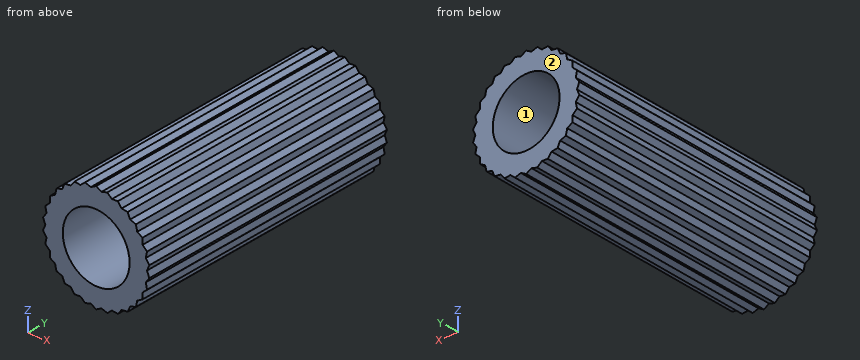
```python
from build123d import *

# Parameters (mm, degrees)
SKETCH_1_R      = 1
EXTRUDE_1_DEPTH = 8


with BuildPart() as part:
    # 草图1 → 凸台-拉伸1 (new body)
    with BuildSketch(Plane(origin=(0, 0, 0), x_dir=(1, 0, 0), z_dir=(0, 1, 0))):
        Polygon((0, 1.6), (-0.158843146, 1.511291584), (-0.332658705, 1.565036161), (-0.469587231, 1.44524089), (-0.650778629, 1.461672732), (-0.7598081, 1.316026234), (-0.940456404, 1.294427191), (-1.01682171, 1.129294916), (-1.189031721, 1.07060897), (-1.229395331, 0.893207992), (-1.385640646, 0.8), (-1.388238477, 0.618083592), (-1.521690426, 0.494427191), (-1.486408941, 0.315945974), (-1.591235033, 0.167245541), (-1.519616201, 0), (-1.591235033, -0.167245541), (-1.486408941, -0.315945974), (-1.521690426, -0.494427191), (-1.388238477, -0.618083592), (-1.385640646, -0.8), (-1.229395331, -0.893207992), (-1.189031721, -1.07060897), (-1.01682171, -1.129294916), (-0.940456404, -1.294427191), (-0.7598081, -1.316026234), (-0.650778629, -1.461672732), (-0.469587231, -1.44524089), (-0.332658705, -1.565036161), (-0.158843146, -1.511291584), (0, -1.6), (0.158843146, -1.511291584), (0.332658705, -1.565036161), (0.469587231, -1.44524089), (0.650778629, -1.461672732), (0.7598081, -1.316026234), (0.940456404, -1.294427191), (1.01682171, -1.129294916), (1.189031721, -1.07060897), (1.229395331, -0.893207992), (1.385640646, -0.8), (1.388238477, -0.618083592), (1.521690426, -0.494427191), (1.486408941, -0.315945974), (1.591235033, -0.167245541), (1.519616201, 0), (1.591235033, 0.167245541), (1.486408941, 0.315945974), (1.521690426, 0.494427191), (1.388238477, 0.618083592), (1.385640646, 0.8), (1.229395331, 0.893207992), (1.189031721, 1.07060897), (1.01682171, 1.129294916), (0.940456404, 1.294427191), (0.7598081, 1.316026234), (0.650778629, 1.461672732), (0.469587231, 1.44524089), (0.332658705, 1.565036161), (0.158843146, 1.511291584), align=None)
        Circle(SKETCH_1_R, mode=Mode.SUBTRACT)
    extrude(amount=EXTRUDE_1_DEPTH)


solid = part.part
```
The listing builds one solid part. Answer for the finished solid, in the listing's coordinates (mm). Face numbers are marked on the shaded views. Coordinates: 2 decimals unless noted, no trailing zeros. Loops run counter-clockwise (first coordinate to the right, second up) from the corner with the lowest first, then second, coordinate; pieces in that order, holes last. Notation, with made-up numbers: (4.25, -2) - (23.25, -2) arc R7 cw to (23.25, 6) - close; hole circle Ø2 at (61, 3.25). An arc over 180 degrees is marked (long way). Write item = value, one per line.
1) Section A-A (z = 0.7) is taken. Determine the outline of the cut face in (x, y).
Responses:
outline = (-1.39, 0) - (-0.71, 0) - (-0.71, 8) - (-1.39, 8) - close; (0.71, 0) - (1.39, 0) - (1.39, 8) - (0.71, 8) - close
2) Determine the mould class of the marked faces 1 and 2 for opening direction Z: pulls with the +Z half, pulls with the -Z half, needs draft (parallel to the pull), parting line crosses it, or undercut.
Responses:
face_1 = undercut
face_2 = needs draft
3) Find the intervals of material crossed by line 1 along Z through (x, y) = (-0.6, 5.25); line 2 along X through (y, z) = (7.25, 0.4); line 3 along X through (y, z) = (5, -1.2), in increasing order.
Responses:
line_1 = -1.46 to -0.8, 0.8 to 1.46
line_2 = -1.5 to -0.92, 0.92 to 1.5
line_3 = -0.98 to 0.98
